```python
from build123d import *

# Parameters (mm, degrees)
SKETCH024_W     = 80
SKETCH024_H     = 110
PAD008_DEPTH    = 2
SKETCH030_W     = 80
SKETCH030_H     = 110
PAD009_DEPTH    = 25
SKETCH029_R     = 1.7
POCKET016_DEPTH = 10
SKETCH031_R     = 3.25
POCKET017_DEPTH = 2.001
FILLET006_R     = 2.9
CHAMFER005_SIZE = 1.3


with BuildPart() as part:
    # Sketch024 → Pad008 (new body)
    with BuildSketch(Plane.XY):
        with Locations((0, 55)):
            Rectangle(SKETCH024_W, SKETCH024_H)
    extrude(amount=PAD008_DEPTH)

    # Sketch030 (on Face6 of Pad008) → Pad009 (join)
    with BuildSketch(Plane.XY.offset(2)):
        with Locations((0, 55)):
            Rectangle(SKETCH030_W, SKETCH030_H)
        Polygon((-38, 102), (-32, 102), (-32, 108), (-14.67, 108), (-14.67, 102), (-8.67, 102), (-8.67, 108), (8.66, 108), (8.66, 102), (14.66, 102), (14.66, 108), (31.99, 108), (31.99, 102), (38, 102), (38, 74.66), (32, 74.66), (32, 68.66), (38, 68.66), (38, 41.33), (32, 41.33), (32, 35.33), (38, 35.33), (38, 8), (32, 8), (32, 2), (14.66, 2), (14.66, 8), (8.66, 8), (8.66, 2), (-8.67, 2), (-8.67, 8), (-14.67, 8), (-14.67, 2), (-32, 2), (-32, 8), (-38, 8), (-38, 35.33), (-32, 35.33), (-32, 41.33), (-38, 41.33), (-38, 68.66), (-32, 68.66), (-32, 74.66), (-38, 74.66), align=None, mode=Mode.SUBTRACT)
    extrude(amount=PAD009_DEPTH)

    # Sketch029 (on Face3 of Pad009) → Pocket016 (cut)
    with BuildSketch(Plane.XY.offset(27)):
        with Locations((-11.667, 5)):
            Circle(SKETCH029_R)
        with Locations((11.666, 5)):
            Circle(SKETCH029_R)
        with Locations((35, 5)):
            Circle(SKETCH029_R)
        with Locations((-35, 38.333)):
            Circle(SKETCH029_R)
        with Locations((-35, 71.666)):
            Circle(SKETCH029_R)
        with Locations((-35, 105)):
            Circle(SKETCH029_R)
        with Locations((35, 38.333)):
            Circle(SKETCH029_R)
        with Locations((35, 71.666)):
            Circle(SKETCH029_R)
        with Locations((35, 105)):
            Circle(SKETCH029_R)
        with Locations((-11.667, 105)):
            Circle(SKETCH029_R)
        with Locations((11.666, 105)):
            Circle(SKETCH029_R)
        with Locations((-35, 5)):
            Circle(SKETCH029_R)
    extrude(amount=-POCKET016_DEPTH, mode=Mode.SUBTRACT)

    # Sketch031 (on Face28 of Pocket016) → Pocket017 (cut, through all)
    with BuildSketch(Plane.XZ.offset(-108)):
        with Locations((0, 14)):
            Circle(SKETCH031_R)
    extrude(amount=-POCKET017_DEPTH, mode=Mode.SUBTRACT)

    # Fillet006
    fillet006_edges = [part.edges().sort_by_distance(p)[0] for p in [
        (-32, 8, 14.5),
        (-14.67, 8, 14.5),
        (-8.67, 8, 14.5),
        (8.66, 8, 14.5),
        (14.66, 8, 14.5),
        (32, 8, 14.5),
        (-32, 35.33, 14.5),
        (-32, 41.33, 14.5),
        (-32, 68.66, 14.5),
        (-32, 74.66, 14.5),
        (32, 35.33, 14.5),
        (32, 41.33, 14.5),
        (32, 68.66, 14.5),
        (32, 74.66, 14.5),
        (31.99, 102, 14.5),
        (14.66, 102, 14.5),
        (8.66, 102, 14.5),
        (-8.67, 102, 14.5),
        (-14.67, 102, 14.5),
        (-32, 102, 14.5),
    ]]
    fillet(fillet006_edges, radius=FILLET006_R)

    # Chamfer005
    chamfer005_edges = [part.edges().sort_by_distance(p)[0] for p in [
        (40, 110, 13.5),
        (-40, 110, 13.5),
        (40, 0, 13.5),
        (-40, 0, 13.5),
    ]]
    chamfer(chamfer005_edges, length=CHAMFER005_SIZE)


solid = part.part
```
Geometry: final body of the model. Coordinates: model frame, mm. Coordinates: 2 decimals unless noted, no trailing zeros. Write each loop counter-clockwise with the first axis right and the second up, starting at its lowest first coordinate (ties: lowest second). Pieces come first, ordered by that corner, then holes. Notation, with made-up numbers: M 24.25,85 L 75.25,85 A23 ccw 75.25,120 Z; hole C -4.5,86 d4. An arc over 180 degrees is marked long. Use CSV: the item, a comma, the result in double quotes. Start each with the question number.
1. Cut plane B-B on x = -19.5. Return the cut outline in (y, z).
2. Mould query, pull axis X, two halves, no side actions, for faces 1 (the face through (14.66, 4, 14)), 2 (the face through (-1, 110, 10)). Classes: pulls with the +X half, pulls with the -X half, needs draft (parallel to the pull), parting line crosses it, or undercut.
3. Ray query, probe 1 along Y at (x, z) = (36, 9.25); probe 2 along Y at (x, z) = (-23, 11); probe 3 along X at (y, z) = (44, 19.5). Return the intervals inside material, ascending.
4. First-contact query: P1, Ø4, axis at x = 32, y = 42.5, coming from the +Z side; P2, Ø1.7, axis at x = 35, y = 72, coming from the +Z side. Flat tips, straight axial feed; report the tip coordinate or a pass-through.
5. Cut plane A-A on y = 92. Return the cut outline in (x, z).
6. Cut plane C-C on z = 24.25. Count the separate pieces of the cut face and the enclosed holes in it, plus the area to 3 significant figures.
Entries:
1,outline,"M 0,0 L 110,0 L 110,27 L 108,27 L 108,2 L 2,2 L 2,27 L 0,27 Z"
2,face 1,"undercut"
2,face 2,"needs draft"
3,probe 1,"0 to 8, 35.33 to 41.33, 68.66 to 74.66, 102 to 110"
3,probe 2,"0 to 2, 108 to 110"
3,probe 3,"-40 to -38, 38 to 40"
4,P1,"z = 2"
4,P2,"z = 17"
5,outline,"M -40,0 L 40,0 L 40,27 L 38,27 L 38,2 L -38,2 L -38,27 L -40,27 Z"
6,separate pieces,"1"
6,enclosed holes,"13"
6,area,"1,030 mm²"
